Autodesk Inventor part; units mm, degrees
ref_plane "Start Plane" through (0, 0, 20) normal (0, 0, 1) x (1, 0, 0)
ref_plane "End Plane" through (0, 0, 680) normal (0, 0, 1) x (1, 0, 0)
ref_plane "YZ Plane" through (0, 0, 0) normal (1, 0, 0) x (0, 1, 0)
ref_plane "Start Plane" through (0, 0, 20) normal (0, 0, 1) x (1, 0, 0)
ref_plane "End Plane" through (0, 0, 680) normal (0, 0, 1) x (1, 0, 0)
sketch "Sketch" plane through (0, 0, 0) normal (0, 0, 1) x (1, 0, 0)
  line L0 (-20, -16) -> (-20, 16)
  line L1 (-16, 20) -> (16, 20)
  line L2 (20, 16) -> (20, -16)
  line L3 (16, -20) -> (-16, -20)
  arc A0 (-20, -16) -> (-16, -20) centre (-16, -16) ccw
  arc A1 (20, 16) -> (16, 20) centre (16, 16) ccw
  arc A2 (-16, 20) -> (-20, 16) centre (-16, 16) ccw
  arc A3 (16, -20) -> (20, -16) centre (16, -16) ccw
  arc A4 (-16, 18) -> (-18, 16) centre (-16, 16) ccw
  line L4 (-16, 18) -> (16, 18)
  arc A5 (18, 16) -> (16, 18) centre (16, 16) ccw
  line L5 (18, 16) -> (18, -16)
  arc A6 (16, -18) -> (18, -16) centre (16, -16) ccw
  line L6 (16, -18) -> (-16, -18)
  arc A7 (-18, -16) -> (-16, -18) centre (-16, -16) ccw
  line L7 (-18, -16) -> (-18, 16)
  line L8 (0, 29.1598) -> (0, -29.1598) construction
  line L9 (-29.1598, 0) -> (29.1598, 0) construction
  dimension "d7" = 4
  dimension "d9" = 40
  dimension "d11" = 40
  dimension "d12" = 2
  dimension "d15" = 20
  dimension "d16" = 20
extrude "Body" add sketch "Sketch" along normal up to surface (660 mm away) from surface at 20
sketch "Sketch3" plane through (0, 0, 0) normal (0, 0, 1) x (1, 0, 0)
  line L0 (0, 0) -> (10, 0)
ref_plane "Work Plane3" through (0, 0, 0) normal (0, -1, 0) x (1, 0, 0)
sketch "Sketch4" plane through (0, 0, 0) normal (0, -1, 0) x (1, 0, 0)
  line L0 (-2, 20) -> (12, 20)
  line L1 (-2, 680) -> (12, 680)
  dimension "d18" = 660
equation "\"d7\" = G_IR"
equation "\"d9\" = G_W"
equation "\"d11\" = G_H"
equation "\"d12\" = G_T"
equation "\"d15\" = 0.5 * d9"
equation "\"d16\" = 0.5 * d11"
equation "\"d3\" = G_L"
equation "\"G_W\" = 40"
equation "\"G_H\" = 40"
equation "\"G_T\" = 2"
equation "\"G_IR\" = 4"
equation "\"G_L\" = d18"
properties part number "ISO 10799-2 - 40x40x2 - 660" material "Steel, Mild"
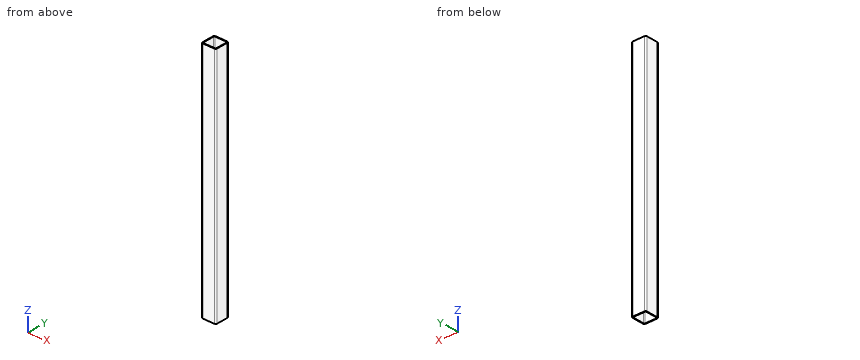
Read the model definition and answer for the solid it produces. Units are mm, in the model's axes. Round coordinates to 2 decimals unless told otherwise and drop trailing zeros. Write each loop counter-clockwise with the first axis right and the second up, starting at its lowest first coordinate (ties: lowest second). Pieces come first, ordered by that corner, then holes.
Q1. Find section B-B on z = 389.5. Determine the outline of the cut face in (x, y), and give its area (3 significant figures).
Values:
outline: (-20, -16) arc R4 ccw to (-16, -20) - (16, -20) arc R4 ccw to (20, -16) - (20, 16) arc R4 ccw to (16, 20) - (-16, 20) arc R4 ccw to (-20, 16) - close; hole (-18, -16) arc R2 ccw to (-16, -18) - (16, -18) arc R2 ccw to (18, -16) - (18, 16) arc R2 ccw to (16, 18) - (-16, 18) arc R2 ccw to (-18, 16) - close
area: 294 mm2
Q2. Find section A-A on y = 9.5. Determine the outline of the cut face in (x, z), and give its area (3 significant figures).
Values:
outline: (-20, 20) - (-18, 20) - (-18, 680) - (-20, 680) - close; (18, 20) - (20, 20) - (20, 680) - (18, 680) - close
area: 2,640 mm2
Q3. Straight lines are drawn through the part: line 1 (X direction, y = -11, z = 275); line 2 (Y direction, x = 16.5, z = 320.5). For each, find the intervals that lie inside material, in ascending order.
Values:
line 1: x = -20 to -18, 18 to 20
line 2: y = -19.97 to -17.94, 17.94 to 19.97
